Check sheet for the modelled part. Datum: model origin and axes. Units: mm. A direction names the side the tool comes from. Round coordinates to 2 decimals unless told otherwise and drop trailing zeros. Write each loop counter-clockwise with the first axis right and the second up, starting at its lowest first coordinate (ties: lowest second). Pieces come first, ordered by that corner, then holes.
Item 1: Depth check by flat-ended pin: pin 1 (2.5 mm diameter, centred on x = -1, z = 306, fed in from -Y); pin 2 (2.5 mm diameter, centred on x = -0.5, z = 302.5, fed in from +Y); pin 3 (2 mm diameter, centred on x = -10, z = 296.5, fed in from -Y). Enter the tip coordinate at first touch or a pass-through.
Item 2: Release check for a two-part mould opening along Y. For faces 3 (the flat face through (3, -3, 293.723)), 4 (the flat face through (-5.84, 3.31, 304.91)), 5 (the conical face through (-5.56, -4.27, 309.43)) record: pulls with the +Y half, pulls with the -Y half, needs draft (parallel to the pull), parting line crosses it, or undercut.
Item 3: Section check A-A, the plane x = 0. Record the cut outline in (y, z).
Item 4: Section check D-D, the plane z = 295. Record the cut outline in (x, y).
Item 5: Section check C-C, the plane z = 308.75. Record the cut outline in (x, y), plus the area to 3 significant figures.
Item 6: Material ranges on line 1 along Z through (x, y) = (5.5, 1.25); line 2 along X through (y, z) = (0, 296); line 3 along X through (y, z) = (-0.25, 301.5), recorded low to high.
Item 7: Section check B-B, the plane z = 300.75. Record the cut outline in (x, y) (3 decimals), plus the area to 3 significant figures.
Item 8: Set-up check for faces 1 (the flat face through (0, -6.712, 305)), 2 (the cylindrical face through (-0.867, 3.905, 296.728)): record each of +Z, -Z, +X, -X, +Y, -Y from which the full face is reachable in a straight line by a thin tool's end or side.
from build123d import *

# Parameters (mm, degrees)
SKETCH057_R     = 4
POCKET022_DEPTH = 25.927831
POCKET023_DEPTH = 14


with BuildPart() as part:
    # Sketch056 → Revolution004 (revolve)
    with BuildSketch(Plane.XZ):
        Polygon((0, 319.649472), (11.88, 302.332844), (14.5, 293.722641), (0, 293.722641), align=None)
    revolve(axis=Axis((0, 0, 0), (0, 0, 1)))

    # Sketch057 (on Face3 of Revolution004) → Pocket022 (cut, through all)
    with BuildSketch(Plane(origin=(0, 0, 293.722641), x_dir=(1, 0, 0), z_dir=(0, 0, -1))):
        Circle(SKETCH057_R)
    extrude(amount=-POCKET022_DEPTH, mode=Mode.SUBTRACT)

    # Sketch058 (on DatumPlane) → Pocket023 (cut)
    with BuildSketch(Plane(origin=(0, 0, 313.818958), x_dir=(0, -1, 0), z_dir=(0, 0, -1))):
        Polygon((6.711697, -3.875), (6.711697, 3.875), (0, 7.75), (-6.711697, 3.875), (-6.711697, -3.875), (0, -7.75), align=None)
    extrude(amount=POCKET023_DEPTH, mode=Mode.SUBTRACT)


solid = part.part
Values found:
1. pin 1: stops at y = -10.18
1. pin 2: stops at y = 12.2
1. pin 3: stops at y = -10.36
2. face 3: needs draft
2. face 4: undercut
2. face 5: parting line crosses it
3. outline: (-14.5, 293.72) - (-4, 293.72) - (-4, 299.82) - (-6.71, 299.82) - (-6.71, 309.87) - (-11.88, 302.33) - close; (4, 293.72) - (14.5, 293.72) - (11.88, 302.33) - (6.71, 309.87) - (6.71, 299.82) - (4, 299.82) - close
4. outline: circle Ø28.22 at (0, 0); hole circle Ø8 at (0, 0)
5. outline: (-7.46, -0.5) arc R7.48 ccw to (-4.16, -6.21) - close; (-7.46, 0.5) - (-4.16, 6.21) arc R7.48 ccw to start; (-3.3, -6.71) arc R7.48 ccw to (3.3, -6.71) - close; (-3.3, 6.71) - (3.3, 6.71) arc R7.48 ccw to start; (4.16, -6.21) arc R7.48 ccw to (7.46, -0.5) - close; (4.16, 6.21) - (7.46, 0.5) arc R7.48 ccw to start
5. area: 20.4 mm2
6. line 1: z = 293.72 to 299.82
6. line 2: x = -13.81 to -4, 4 to 13.81
6. line 3: x = -12.13 to -7.61, 7.61 to 12.13
7. outline: circle Ø24.723 at (0, 0); hole (-7.75, 0) - (-3.875, -6.712) - (3.875, -6.712) - (7.75, 0) - (3.875, 6.712) - (-3.875, 6.712) - close
7. area: 324 mm2
8. face 1: +Z
8. face 2: +Z, -Z
